Design review of the part built by this model. Coordinates are the model's own, in mm. Give positions to 0.01 mm unless a question says otherwise; leave off trailing zeros. Order: outer loops, then holes, each group sorted by start corner. A loop starts at its lowest first (then second) coordinate and runs counter-clockwise, first axis right, second up. Notation, with made-up numbers: (23, -2.5) -> (30, -2.5) arc R16 cw to (30, 10.5) -> close; hole circle Ø10 at (13.25, 55). An arc over 180 degrees is marked (long way). Return JSON: item names as keys, results as strings.
Autodesk Inventor part; units mm, degrees
ref_plane "YZ Plane" through (0, 0, 0) normal (1, 0, 0) x (0, 1, 0)
ref_plane "XZ Plane" through (0, 0, 0) normal (0, 1, 0) x (-1, 0, 0)
ref_plane "XY Plane" through (0, 0, 0) normal (0, 0, 1) x (1, 0, 0)
sketch "Sketch1" plane through (0, 0, 0) normal (0, 0, 1) x (1, 0, 0)
  line L0 (0, 0) -> (25.4, 0)
  line L1 (25.4, 0) -> (25.4, 25.4)
  line L2 (25.4, 25.4) -> (0, 25.4)
  line L3 (0, 25.4) -> (0, 0)
  line L4 (23.114, 2.286) -> (2.286, 2.286)
  line L5 (2.286, 2.286) -> (2.286, 23.114)
  line L6 (2.286, 23.114) -> (23.114, 23.114)
  line L7 (23.114, 23.114) -> (23.114, 2.286)
  dimension "d0" = 25.4
  dimension "d1" = 25.4
  dimension "d2" = 2.286
extrude "Extrusion1" add sketch "Sketch1" along normal blind 863.6
sketch "Sketch2" plane through (25.4, 0, 0) normal (1, 0, 0) x (0, 0, -1)
  circle A0 centre (-12.7, 12.7) radius 2.5527
  line L0 (0, 25.4) -> (-863.6, 25.4)
  line L1 (0, 0) -> (0, 25.4)
  circle A1 centre (-38.1, 12.7) radius 2.5527
  circle A2 centre (-63.5, 12.7) radius 2.5527
  circle A3 centre (-88.9, 12.7) radius 2.5527
  circle A4 centre (-114.3, 12.7) radius 2.5527
  circle A5 centre (-139.7, 12.7) radius 2.5527
  circle A6 centre (-165.1, 12.7) radius 2.5527
  circle A7 centre (-190.5, 12.7) radius 2.5527
  circle A8 centre (-215.9, 12.7) radius 2.5527
  circle A9 centre (-241.3, 12.7) radius 2.5527
  circle A10 centre (-266.7, 12.7) radius 2.5527
  circle A11 centre (-292.1, 12.7) radius 2.5527
  circle A12 centre (-317.5, 12.7) radius 2.5527
  circle A13 centre (-342.9, 12.7) radius 2.5527
  circle A14 centre (-368.3, 12.7) radius 2.5527
  circle A15 centre (-393.7, 12.7) radius 2.5527
  circle A16 centre (-419.1, 12.7) radius 2.5527
  circle A17 centre (-444.5, 12.7) radius 2.5527
  circle A18 centre (-469.9, 12.7) radius 2.5527
  circle A19 centre (-495.3, 12.7) radius 2.5527
  circle A20 centre (-520.7, 12.7) radius 2.5527
  circle A21 centre (-546.1, 12.7) radius 2.5527
  circle A22 centre (-571.5, 12.7) radius 2.5527
  circle A23 centre (-596.9, 12.7) radius 2.5527
  circle A24 centre (-622.3, 12.7) radius 2.5527
  circle A25 centre (-647.7, 12.7) radius 2.5527
  circle A26 centre (-673.1, 12.7) radius 2.5527
  circle A27 centre (-698.5, 12.7) radius 2.5527
  circle A28 centre (-723.9, 12.7) radius 2.5527
  circle A29 centre (-749.3, 12.7) radius 2.5527
  circle A30 centre (-774.7, 12.7) radius 2.5527
  circle A31 centre (-800.1, 12.7) radius 2.5527
  circle A32 centre (-825.5, 12.7) radius 2.5527
  circle A33 centre (-850.9, 12.7) radius 2.5527
  point P0 (0, 12.7)
  dimension "d5" = 5.1054
  dimension "d6" = 12.7
  dimension "d7" = 12.7
  dimension "d10" = 25.4
extrude "Extrusion2" cut sketch "Sketch2" against normal through all
properties part number "Angled_bar" material "Aluminum 6061"
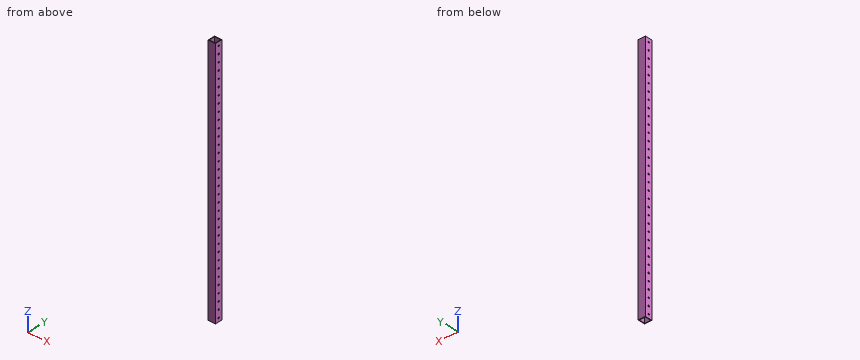
Item 1: Wall thickness on L1, parallel to Y at x = 20, z = 629.5; L2, parallel to Y at x = 1.75, z = 88.9: over which ranges is each line inside the solid? List them lowest first. Write a range as [from, to].
Result set:
{"L1": "y = [0, 2.29], [23.11, 25.4]", "L2": "y = [0, 10.15], [15.25, 25.4]"}
Item 2: Add section A-A (x = 11.5). Give the boundary of the cut face in (y, z).
Result set:
{"outline": "(0, 0) -> (2.29, 0) -> (2.29, 863.6) -> (0, 863.6) -> close; (23.11, 0) -> (25.4, 0) -> (25.4, 863.6) -> (23.11, 863.6) -> close"}
Item 3: For pin 1 (3 mm diameter, centred on y = 12.7, z = 215.9, fed in from +X), flat-tipped, find the tip position at first contact; note if it passes through.
Result set:
{"pin 1": "passes through"}
